Autodesk Inventor part; units mm, degrees
ref_plane "YZ Plane" through (0, 0, 0) normal (1, 0, 0) x (0, 1, 0)
ref_plane "XZ Plane" through (0, 0, 0) normal (0, 1, 0) x (-1, 0, 0)
ref_plane "XY Plane" through (0, 0, 0) normal (0, 0, 1) x (1, 0, 0)
sketch "Sketch1" plane through (0, 0, 0) normal (0, 0, 1) x (1, 0, 0)
  line L0 (0, 0) -> (-25.4, 0)
  line L1 (-25.4, 0) -> (-25.4, -50.8)
  line L2 (-25.4, -50.8) -> (0, -50.8)
  line L3 (0, -50.8) -> (0, 0)
  line L4 (-22.225, -3.175) -> (-3.175, -3.175)
  line L5 (-3.175, -3.175) -> (-3.175, -47.625)
  line L6 (-3.175, -47.625) -> (-22.225, -47.625)
  line L7 (-22.225, -47.625) -> (-22.225, -3.175)
  dimension "d0" = 25.4
  dimension "d1" = 50.8
  dimension "d2" = 3.175
extrude "Extrusion1" add sketch "Sketch1" along normal blind 165.1
sketch "Sketch2" plane through (0, -50.8, 0) normal (1, 0, 0) x (0, 0, -1)
  circle A0 centre (-25.4, 25.4) radius 14.2875
  line L0 (0, 0) -> (0, 50.8)
  line L1 (0, 50.8) -> (-165.1, 50.8)
  circle A1 centre (-139.7, 25.4) radius 14.2875
  line L2 (0, 0) -> (-165.1, 0)
  line L3 (-165.1, 0) -> (-165.1, 50.8)
  dimension "d5" = 28.575
  dimension "d6" = 25.4
  dimension "d7" = 25.4
  dimension "d8" = 28.575
  dimension "d9" = 25.4
  dimension "d10" = 25.4
extrude "Extrusion2" cut sketch "Sketch2" against normal blind 177.8 contours A0 | A1
properties part number "intake srms"
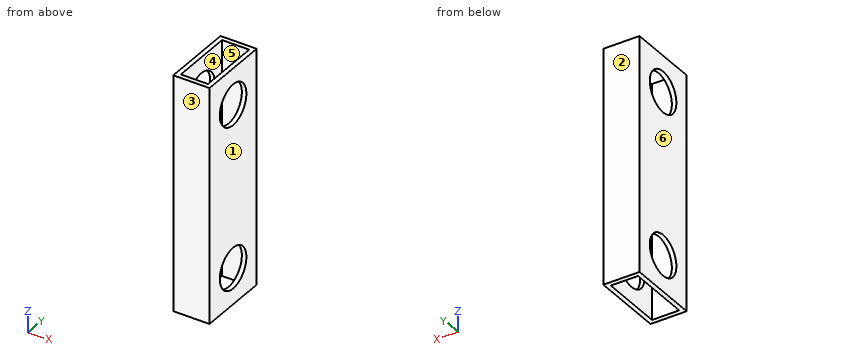
CAD build for the part. Positions are in the model's coordinates, mm. Face numbers are marked on the shaded views. A direction names the side the tool comes from. Round coordinates to 2 decimals unless told otherwise and drop trailing zeros. Write each loop counter-clockwise with the first axis right and the second up, starting at its lowest first coordinate (ties: lowest second). Pieces come first, ordered by that corner, then holes. Notation, with made-up numbers: M 78.25,71 L 96.25,71 A20 ccw 96.25,90 Z; hole C 40.5,-37.5 d10. An arc over 180 degrees is marked long. Put each result on its own line as item: value. Start each with the question number.
1) Saw through at D-D, the plane z = 63. Write the cut outline in (x, y) (3 decimals), and give its area (3 significant figures).
2) Pin check, flat tip, straight feed: pin 1 Ø3 at (x, y) = (-20, -10.5) entering from +Z. Stop position of the tip, or through.
3) Saw through at C-C, the plane x = -19.75. Write the cut outline in (y, z) (3 decimals).
4) Pull direction Y, two halves, no side cores. Call the marked faces 1, 2, 3 and 4: pulls with the +Y half, pulls with the -Y half, needs draft (parallel to the pull), parting line crosses it, or undercut.
5) 3-axis set-ups, long thin cutter, end or side, ignore diameter. For the marked faces 5 and 6: which of +Z, -Z, +X, -X, +Y, -Y reach the whole face in a straight line?
6) Saw through at A-A, the plane y = -25.4. Write the cut outline in (x, z) (1 decimal), and give its area (3 significant figures).
7) Saw through at B-B, the plane z = 25.4. Write the cut outline in (x, y) (1 decimal), and give its area (3 significant figures).
8) Drill centre lines: probe 1 along X at (y, z) = (-39.5, 89) (3 decimals); probe 2 along Y at (x, z) = (-19, 75.5) (3 decimals); probe 3 along Y at (x, z) = (-22.9, 25.4). Where is each one in solid material? Low to high. Write a range as [from, to].
Resolved:
1. outline: M -25.4,-50.8 L 0,-50.8 L 0,0 L -25.4,0 Z; hole M -22.225,-47.625 L -3.175,-47.625 L -3.175,-3.175 L -22.225,-3.175 Z
1. area: 444 mm²
2. pin 1: through
3. outline: M -50.8,0 L -47.625,0 L -47.625,165.1 L -50.8,165.1 Z; M -3.175,0 L 0,0 L 0,165.1 L -3.175,165.1 Z
4. face 1: needs draft
4. face 2: pulls with the +Y half
4. face 3: pulls with the -Y half
4. face 4: undercut
5. face 5: +Z, -Z
5. face 6: +Z, -Z, -X, +Y, -Y
6. outline: M -25.4,0 L -22.2,0 L -22.2,11.1 L -25.4,11.1 Z; M -25.4,39.7 L -22.2,39.7 L -22.2,125.4 L -25.4,125.4 Z; M -25.4,154 L -22.2,154 L -22.2,165.1 L -25.4,165.1 Z; M -3.2,0 L 0,0 L 0,11.1 L -3.2,11.1 Z; M -3.2,39.7 L 0,39.7 L 0,125.4 L -3.2,125.4 Z; M -3.2,154 L 0,154 L 0,165.1 L -3.2,165.1 Z
6. area: 685 mm²
7. outline: M -25.4,-50.8 L 0,-50.8 L 0,-39.7 L -3.2,-39.7 L -3.2,-47.6 L -22.2,-47.6 L -22.2,-39.7 L -25.4,-39.7 Z; M -25.4,-11.1 L -22.2,-11.1 L -22.2,-3.2 L -3.2,-3.2 L -3.2,-11.1 L 0,-11.1 L 0,0 L -25.4,0 Z
7. area: 262 mm²
8. probe 1: [-25.4, -22.225], [-3.175, 0]
8. probe 2: [-50.8, -47.625], [-3.175, 0]
8. probe 3: [-50.8, -39.69], [-11.11, 0]
